from build123d import *

# Parameters (mm, degrees)
SKETCH1_W           = 20.6248
SKETCH1_H           = 20.6248
BOSS_EXTRUDE1_DEPTH = 1.5875
CHAMFER1_SIZE       = 2.54
SKETCH2_R           = 1.524
CUT_EXTRUDE1_DEPTH  = 15.670083291


with BuildPart() as part:
    # Sketch1 → Boss-Extrude1 (new body)
    with BuildSketch(Plane(origin=(0, 0, 0), x_dir=(1, 0, 0), z_dir=(0, 1, 0))):
        Rectangle(SKETCH1_W, SKETCH1_H)
    extrude(amount=BOSS_EXTRUDE1_DEPTH)

    # Chamfer1
    chamfer1_edges = [part.edges().sort_by_distance(p)[0] for p in [
        (10.3124, 0.79375, 10.3124),
        (-10.3124, 0.79375, 10.3124),
        (-10.3124, 0.79375, -10.3124),
        (10.3124, 0.79375, -10.3124),
    ]]
    chamfer(chamfer1_edges, length=CHAMFER1_SIZE)

    # Sketch2 → Cut-Extrude1 (cut, through all)
    with BuildSketch(Plane(origin=(0, 1.5875, 0), x_dir=(1, 0, 0), z_dir=(0, 1, 0))):
        with Locations(Location((-7.5438, 7.5438, 0), (0, 0, 270))):
            Circle(SKETCH2_R)
        with Locations(Location((7.5438, 7.5438, 0), (0, 0, 270))):
            Circle(SKETCH2_R)
        with Locations(Location((7.5438, -7.5438, 0), (0, 0, 270))):
            Circle(SKETCH2_R)
        with Locations(Location((-7.5438, -7.5438, 0), (0, 0, 270))):
            Circle(SKETCH2_R)
    extrude(amount=-CUT_EXTRUDE1_DEPTH, mode=Mode.SUBTRACT)


solid = part.part
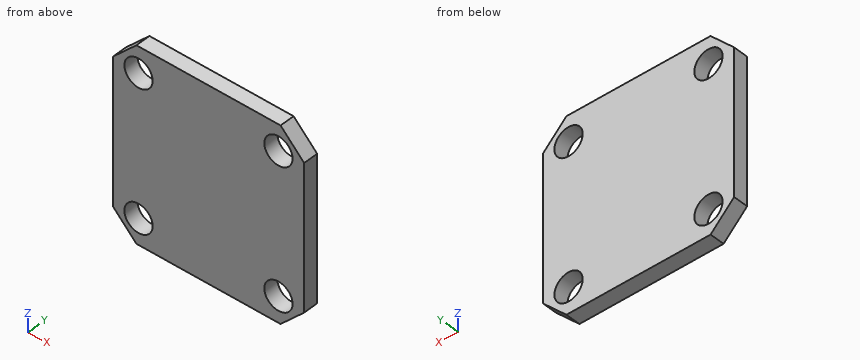
Check sheet for the modelled part. Datum: model origin and axes. Units: mm. Coordinates: 2 decimals unless noted, no trailing zeros. Loops run counter-clockwise (first coordinate to the right, second up) from the corner with the lowest first, then second, coordinate; pieces in that order, holes last. Notation, with made-up numbers: (30.5, 28) -> (54.5, 28) arc R17 cw to (54.5, 43) -> close; hole circle Ø5 at (25, -13.75). An arc over 180 degrees is marked (long way). Write item = value, one per line. Start each with the question number.
1. Section check B-B on x = 6.75. Record the cut outline in (y, z), then the cut area to 3 significant figures.
2. Section check A-A on z = -8.5. Record the cut outline in (x, y).
3. Section check C-C on y = 0.8. Record the cut outline in (x, z), then the cut area to 3 significant figures.
4. Material ranges on line 1 (X direction, y = 0.3, z = -7.5); line 2 (X direction, y = 1.3, z = -7.25); line 3 (Z direction, x = 7, y = 0.55), recorded low to high.
Responses:
q1.outline = (0, -10.31) -> (1.59, -10.31) -> (1.59, -8.84) -> (0, -8.84) -> close; (0, -6.24) -> (1.59, -6.24) -> (1.59, 6.24) -> (0, 6.24) -> close; (0, 8.84) -> (1.59, 8.84) -> (1.59, 10.31) -> (0, 10.31) -> close
q1.area = 24.5 mm2
q2.outline = (-9.58, 0) -> (-8.73, 0) -> (-8.73, 1.59) -> (-9.58, 1.59) -> close; (-6.36, 0) -> (6.36, 0) -> (6.36, 1.59) -> (-6.36, 1.59) -> close; (8.73, 0) -> (9.58, 0) -> (9.58, 1.59) -> (8.73, 1.59) -> close
q3.outline = (-10.31, -7.77) -> (-7.77, -10.31) -> (7.77, -10.31) -> (10.31, -7.77) -> (10.31, 7.77) -> (7.77, 10.31) -> (-7.77, 10.31) -> (-10.31, 7.77) -> close; hole circle Ø3.05 at (-7.54, -7.54); hole circle Ø3.05 at (-7.54, 7.54); hole circle Ø3.05 at (7.54, -7.54); hole circle Ø3.05 at (7.54, 7.54)
q3.area = 383 mm2
q4.line_1 = -10.31 to -9.07, -6.02 to 6.02, 9.07 to 10.31
q4.line_2 = -10.31 to -9.04, -6.05 to 6.05, 9.04 to 10.31
q4.line_3 = -10.31 to -8.97, -6.12 to 6.12, 8.97 to 10.31
